Read the model definition and answer for the solid it produces. Units are mm, in the model's axes. Face numbers are marked on the shaded views. A direction names the side the tool comes from. Coordinates: 2 decimals unless noted, no trailing zeros. Loops run counter-clockwise (first coordinate to the right, second up) from the corner with the lowest first, then second, coordinate; pieces in that order, holes last. Notation, with made-up numbers: (76.5, -15) - (107.5, -15) arc R23 ccw to (107.5, 19) - close; hole circle Ø9 at (-18.5, 36.5). An arc over 180 degrees is marked (long way). Use CSV: the item, a comma, the result in double quotes.
```python
from build123d import *

# Parameters (mm, degrees)
BODY_DEPTH                             = 45
BOTTOM_TRIM_SIZE                       = 30
BOTTOM_TRIM_SIZE2                      = 42.426406871
FRONT_MOUNTING_HOLES_REACH             = 92
SKETCH2_R                              = 4.3
SKETCH2_R_2                            = 1.6
FRONT_MOUNTING_HOLES_COUNTERBORE_DEPTH = 3.5
BACK_MOUNTING_SLOT_REACH               = 92


with BuildPart() as part:
    # Sketch1 → Body (new body)
    with BuildSketch(Plane.XY):
        with BuildLine():
            Line((0, 0), (0, 191.213203436))
            Line((0, 191.213203436), (80, 191.213203436))
            ThreePointArc((80, 191.213203436), (87.071067812, 188.284271247), (90, 181.213203436))
            Line((90, 181.213203436), (90, 94.142135624))
            ThreePointArc((90, 94.142135624), (89.238795325, 90.3153013), (87.071067812, 87.071067812))
            Line((87.071067812, 87.071067812), (0, 0))
        make_face()
        with BuildLine():
            Line((72.071067812, 93.284271247), (28.656854249, 49.870057685))
            ThreePointArc((28.656854249, 49.870057685), (19.938532541, 48.135875674), (15, 55.526911935))
            Line((15, 55.526911935), (15, 168.213203436))
            ThreePointArc((15, 168.213203436), (17.343145751, 173.870057685), (23, 176.213203436))
            Line((23, 176.213203436), (65, 176.213203436))
            ThreePointArc((65, 176.213203436), (72.071067812, 173.284271247), (75, 166.213203436))
            Line((75, 166.213203436), (75, 100.355339059))
            ThreePointArc((75, 100.355339059), (74.238795325, 96.528504736), (72.071067812, 93.284271247))
        make_face(mode=Mode.SUBTRACT)
    extrude(amount=BODY_DEPTH)

    # Bottom Trim
    bottom_trim_edges = [part.edges().sort_by_distance(p)[0] for p in [
        (0, 0, 22.5),
    ]]
    bottom_trim_side = [part.faces().sort_by_distance(p)[0] for p in [
        (0, 95.606601718, 22.5),
    ]]
    chamfer(bottom_trim_edges, length=BOTTOM_TRIM_SIZE, length2=BOTTOM_TRIM_SIZE2, reference=bottom_trim_side[0])

    # Sketch2 → Front Mounting Holes (cut, up to next)
    with BuildSketch(Plane(origin=(90, 0, 0), x_dir=(0, 0, -1), z_dir=(1, 0, 0)), mode=Mode.PRIVATE) as front_mounting_holes_sk1:
        with Locations((-22.5, 137.67766953)):
            Circle(SKETCH2_R)
    front_mounting_holes_tool1 = extrude(front_mounting_holes_sk1.sketch, amount=-FRONT_MOUNTING_HOLES_REACH, mode=Mode.PRIVATE) & part.part
    add(front_mounting_holes_tool1.solids().sort_by_distance((90, 137.67767, 22.5))[0], mode=Mode.SUBTRACT)
    # Sketch2 → Front Mounting Holes (cut, up to next)
    with BuildSketch(Plane(origin=(90, 0, 0), x_dir=(0, 0, -1), z_dir=(1, 0, 0)), mode=Mode.PRIVATE) as front_mounting_holes_sk2:
        with Locations((-22.5, 152.67766953)):
            Circle(SKETCH2_R_2)
    front_mounting_holes_tool2 = extrude(front_mounting_holes_sk2.sketch, amount=-FRONT_MOUNTING_HOLES_REACH, mode=Mode.PRIVATE) & part.part
    add(front_mounting_holes_tool2.solids().sort_by_distance((90, 152.67767, 22.5))[0], mode=Mode.SUBTRACT)
    # Sketch2 → Front Mounting Holes (cut, up to next)
    with BuildSketch(Plane(origin=(90, 0, 0), x_dir=(0, 0, -1), z_dir=(1, 0, 0)), mode=Mode.PRIVATE) as front_mounting_holes_sk3:
        with Locations((-7.5, 137.67766953)):
            Circle(SKETCH2_R_2)
    front_mounting_holes_tool3 = extrude(front_mounting_holes_sk3.sketch, amount=-FRONT_MOUNTING_HOLES_REACH, mode=Mode.PRIVATE) & part.part
    add(front_mounting_holes_tool3.solids().sort_by_distance((90, 137.67767, 7.5))[0], mode=Mode.SUBTRACT)
    # Sketch2 → Front Mounting Holes (cut, up to next)
    with BuildSketch(Plane(origin=(90, 0, 0), x_dir=(0, 0, -1), z_dir=(1, 0, 0)), mode=Mode.PRIVATE) as front_mounting_holes_sk4:
        with Locations((-22.5, 122.67766953)):
            Circle(SKETCH2_R_2)
    front_mounting_holes_tool4 = extrude(front_mounting_holes_sk4.sketch, amount=-FRONT_MOUNTING_HOLES_REACH, mode=Mode.PRIVATE) & part.part
    add(front_mounting_holes_tool4.solids().sort_by_distance((90, 122.67767, 22.5))[0], mode=Mode.SUBTRACT)
    # Sketch2 → Front Mounting Holes (cut, up to next)
    with BuildSketch(Plane(origin=(90, 0, 0), x_dir=(0, 0, -1), z_dir=(1, 0, 0)), mode=Mode.PRIVATE) as front_mounting_holes_sk5:
        with Locations((-37.5, 137.67766953)):
            Circle(SKETCH2_R_2)
    front_mounting_holes_tool5 = extrude(front_mounting_holes_sk5.sketch, amount=-FRONT_MOUNTING_HOLES_REACH, mode=Mode.PRIVATE) & part.part
    add(front_mounting_holes_tool5.solids().sort_by_distance((90, 137.67767, 37.5))[0], mode=Mode.SUBTRACT)

    # Sketch3 → Front Mounting Holes Counterbore (cut)
    with BuildSketch(Plane.ZY.offset(-75)):
        Polygon((40.35, 136.032221262), (40.35, 139.323117797), (37.5, 140.968566064), (34.65, 139.323117797), (34.65, 136.032221262), (37.5, 134.386772995), align=None)
        Polygon((24.145448267, 155.52766953), (20.854551733, 155.52766953), (19.209103466, 152.67766953), (20.854551733, 149.82766953), (24.145448267, 149.82766953), (25.790896534, 152.67766953), align=None)
        Polygon((20.854551733, 119.82766953), (24.145448267, 119.82766953), (25.790896534, 122.67766953), (24.145448267, 125.52766953), (20.854551733, 125.52766953), (19.209103466, 122.67766953), align=None)
        Polygon((4.65, 139.323117797), (4.65, 136.032221262), (7.5, 134.386772995), (10.35, 136.032221262), (10.35, 139.323117797), (7.5, 140.968566064), align=None)
    extrude(amount=-FRONT_MOUNTING_HOLES_COUNTERBORE_DEPTH, mode=Mode.SUBTRACT)

    # Sketch4 → Back Mounting Slot (cut, up to next)
    with BuildSketch(Plane.ZY, mode=Mode.PRIVATE) as back_mounting_slot_sk1:
        with BuildLine():
            Line((26.6, 161.870057685), (26.6, 61.870057685))
            ThreePointArc((26.6, 61.870057685), (22.5, 57.770057685), (18.4, 61.870057685))
            Line((18.4, 61.870057685), (18.4, 161.870057685))
            ThreePointArc((18.4, 161.870057685), (22.5, 165.970057685), (26.6, 161.870057685))
        make_face()
    back_mounting_slot_tool1 = extrude(back_mounting_slot_sk1.sketch, amount=-BACK_MOUNTING_SLOT_REACH, mode=Mode.PRIVATE) & part.part
    add(back_mounting_slot_tool1.solids().sort_by_distance((0, 111.870058, 22.5))[0], mode=Mode.SUBTRACT)


solid = part.part
```
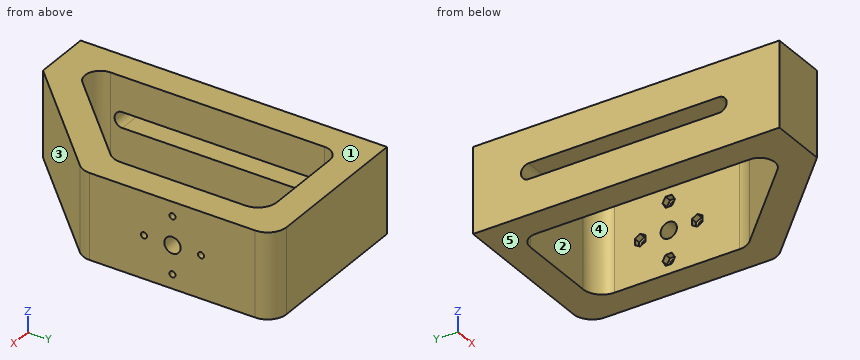
Q1. For a pull along Y with two mould halves and no side action, classify the marked faces 3, 4 and 5 as +Y half, -Y half, draft (parallel to the pull), parting line (faces both ways), or undercut.
Reported:
face 3,"-Y half"
face 4,"undercut"
face 5,"draft"
Q2. The part is cut by section A-A on z = 32.5. Determine the outline of the cut face in (x, y).
Reported:
outline,"(0, 30) - (30, 30) - (87.07, 87.07) arc R10 ccw to (90, 94.14) - (90, 181.21) arc R10 ccw to (80, 191.21) - (0, 191.21) - close; hole (15, 55.53) arc R8 ccw to (28.66, 49.87) - (72.07, 93.28) arc R10 ccw to (75, 100.36) - (75, 166.21) arc R10 ccw to (65, 176.21) - (23, 176.21) arc R8 ccw to (15, 168.21) - close"
Q3. A tool of negligible diameter and unlimited length cuts with its end or side. For the marked faces 1 and 2, from which of +Z, -Z, +X, -X, +Y, -Y can it reach the whole face along a straight path? Write none if from no direction.
Reported:
face 1,"+Z, +X, -X, +Y, -Y"
face 2,"+Z, -Z"
Q4. Find the intervals of material crossed by probe 1 along Z at (x, y) = (13, 66); probe 2 along Y at (x, z) = (80, 22.5); probe 3 along X at (y, z) = (127.5, 17), in increasing order. Write a range as [from, to].
Reported:
probe 1,"z = [0, 18.4], [26.6, 45]"
probe 2,"y = [80, 121.08], [124.28, 133.38], [141.98, 151.08], [154.28, 191.21]"
probe 3,"x = [0, 15], [75, 90]"
Q5. The part is cut by section B-B on x = 10.5. Determine the outline of the cut face in (y, z), and give its area (3 significant figures).
Reported:
outline,"(30, 0) - (191.21, 0) - (191.21, 45) - (30, 45) - close; hole (61.87, 18.4) - (161.87, 18.4) arc R4.1 ccw to (161.87, 26.6) - (61.87, 26.6) arc R4.1 ccw to start"
area,"6,380 mm²"
Q6. The part is cut by section C-C on x = 25. Determine the outline of the cut face in (y, z), and give its area (3 significant figures).
Reported:
outline,"(30, 0) - (47.78, 0) - (47.78, 45) - (30, 45) - close; (176.21, 0) - (191.21, 0) - (191.21, 45) - (176.21, 45) - close"
area,"1,480 mm²"
Q7. Given P1, Ø3.5, axis at x = 76.5, z = 22.5, coming from the -Y side; P2, Ø1.5, axis at y = 65, z = 22.5, coming from the +X side; P3, Ø3, axis at y = 123, z = 21.5, coming from the -X side, each flat-ended and moving along its own axis, determine where each tip first touches the part or whether it passes through.
Reported:
P1,"stops at y = 74.75"
P2,"stops at x = 65.75"
P3,"stops at x = 78.5"
Q8. The part is cut by section D-D on y = 81. Determine the outline of the cut face in (x, z).
Reported:
outline,"(0, 0) - (15, 0) - (15, 18.4) - (0, 18.4) - close; (0, 26.6) - (15, 26.6) - (15, 45) - (0, 45) - close; (59.79, 0) - (81, 0) - (81, 45) - (59.79, 45) - close"
